Work out the finished part from the listing and answer in its coordinate system (mm). Coordinates: 2 decimals unless noted, no trailing zeros. Order: outer loops, then holes, each group sorted by start corner. A loop starts at its lowest first (then second) coordinate and runs counter-clockwise, first axis right, second up. Notation, with made-up numbers: M 0.5,-28 L 34.5,-28 A31 cw 34.5,4 Z; hole C -33.75,-3 d3. An arc over 180 degrees is marked long. Use a Markdown table: item, result.
Autodesk Inventor part; units mm, degrees
ref_plane "YZ Plane" through (0, 0, 0) normal (1, 0, 0) x (0, 1, 0)
ref_plane "XZ Plane" through (0, 0, 0) normal (0, 1, 0) x (-1, 0, 0)
ref_plane "XY Plane" through (0, 0, 0) normal (0, 0, 1) x (1, 0, 0)
sketch "Sketch1" plane through (0, 0, 0) normal (0, 0, 1) x (1, 0, 0)
  circle A0 centre (0, 0) radius 15.875
extrude "Extrusion1" add sketch "Sketch1" along normal blind 6.35
sketch "Sketch3" plane through (0, 0, 6.35) normal (0, 0, 1) x (1, 0, 0)
  circle A0 centre (0, 0) radius 15.875
  circle A1 centre (0, 12.7) radius 1.5875
  circle A2 centre (0, 6.35) radius 1.5875
  circle A3 centre (0, 0) radius 1.5875
  dimension "d4" = 3.175
  dimension "d5" = 3.175
  dimension "d6" = 3.175
  dimension "d7" = 6.35
  dimension "d8" = 6.35
extrude "Extrusion3" cut sketch "Sketch3" against normal blind 6.35 contours A1 | A2 | A3
pattern_circular "Circular Pattern1" count 8 over 360 about axis through (0, 0, 0) along (0, 0, 1) of "Extrusion3"
properties part number "lid"
1. Flat-ended cylindrical pins translate along their axes: P1, Ø3, axis at x = -4.5, z = 3.5, coming from the -Y side; P2, Ø1, axis at y = -5.5, z = 4.5, coming from the -X side; P3, Ø3, axis at y = -9.5, z = 3.5, coming from the -X side. Find the tip coordinate at first contact, or state that the pin passes through.
Answers below:
| item | result |
|---|---|
| P1 | y = -15.59 |
| P2 | x = -15.07 |
| P3 | x = -13.71 |
2. Section B-B on y = -12 is taken. Determine the outline of the cut face in (x, z).
Answers below:
| item | result |
|---|---|
| outline | M -10.39,0 L -1.42,0 L -1.42,6.35 L -10.39,6.35 Z; M 1.42,0 L 10.39,0 L 10.39,6.35 L 1.42,6.35 Z |
3. Section A-A on y = 0 is taken. Give the number of separate pieces and of enclosed holes in the cut face, then the cut area to 3 significant figures.
Answers below:
| item | result |
|---|---|
| separate pieces | 6 |
| enclosed holes | 0 |
| area | 101 mm² |
4. For a pull along Y with two mould halves and no side action, classify faces 1 (the face through (3, 0, 0)), 2 (the face through (14.274, 0.207, 3.219)), 3 (the face through (-3.441, 15.497, 3.131)) as +Y half, -Y half, draft (parallel to the pull), parting line (faces both ways), or undercut.
Answers below:
| item | result |
|---|---|
| face 1 | draft |
| face 2 | undercut |
| face 3 | parting line |
5. Find the intervals of material crossed by probe 1 along Y at (x, z) = (9, 0.75); probe 2 along Y at (x, z) = (0.5, 3); probe 3 along Y at (x, z) = (3.5, 5.75), in increasing order.
Answers below:
| item | result |
|---|---|
| probe 1 | -13.08 to -10.57, -7.39 to 7.39, 10.57 to 13.08 |
| probe 2 | -15.87 to -14.21, -11.19 to -7.86, -4.84 to -1.51, 1.51 to 4.84, 7.86 to 11.19, 14.21 to 15.87 |
| probe 3 | -15.48 to -5.73, -3.25 to 3.25, 5.73 to 15.48 |
